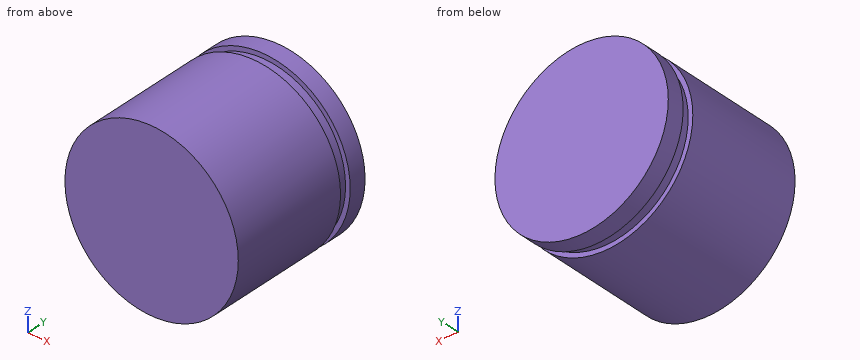
```python
from build123d import *

# Parameters (mm, degrees)
SKETCH1_R           = 7.5
BOSS_EXTRUDE1_DEPTH = 13
SKETCH2_R           = 7.0993
CUT_EXTRUDE1_DEPTH  = 0.9906


with BuildPart() as part:
    # Sketch1 → Boss-Extrude1 (new body)
    with BuildSketch(Plane(origin=(0, 0, 0), x_dir=(1, 0, 0), z_dir=(0, 1, 0))):
        Circle(SKETCH1_R)
    extrude(amount=BOSS_EXTRUDE1_DEPTH)

    # Sketch2 → Cut-Extrude1 (cut)
    with BuildSketch(Plane(origin=(0, 11.476, 0), x_dir=(1, 0, 0), z_dir=(0, 1, 0))):
        Polygon((-10.537332024, 10.483478538), (-10.860452938, -10.950208747), (14.271173695, -10.950208747), (12.440155183, 11.524645927), align=None)
        Circle(SKETCH2_R, mode=Mode.SUBTRACT)
    extrude(amount=-CUT_EXTRUDE1_DEPTH, mode=Mode.SUBTRACT)


solid = part.part
```
Read the model definition and answer for the solid it produces. Units are mm, in the model's axes. Coordinates: 2 decimals unless noted, no trailing zeros. Loops run counter-clockwise (first coordinate to the right, second up) from the corner with the lowest first, then second, coordinate; pieces in that order, holes last.
(1) Flat-ended cylindrical pins translate along their axes: pin 1 Ø3 at (x, y) = (-3, 2) entering from +Z; pin 2 Ø2 at (x, y) = (5.5, 3.5) entering from +Z; pin 3 Ø1 at (x, z) = (-6, 6) entering from +Y; pin 4 Ø5 at (x, y) = (-3, 4) entering from +Z. Find the tip coordinate at first contact, or state that the pin passes through.
Solution:
pin 1: stops at z = 7.35
pin 2: stops at z = 6
pin 3: passes through
pin 4: stops at z = 7.48
(2) The part is cut by section C-C (y = 12.25). Determine the outline of the cut face in (x, z).
Solution:
outline: circle Ø15 at (0, 0)
(3) Consider line 1 along Y through (x, z) = (-5, -5.5); line 2 along X through (y, z) = (4.75, 0.25); line 3 along Z through (x, y) = (-6, 0.5). Determine where each line is inside the solid, lowest interval first.
Solution:
line 1: y = 0 to 10.49, 11.48 to 13
line 2: x = -7.5 to 7.5
line 3: z = -4.5 to 4.5
(4) The part is cut by section B-B (x = 4). Determine the outline of the cut face in (y, z).
Solution:
outline: (0, -6.34) - (10.49, -6.34) - (10.49, -5.87) - (11.48, -5.87) - (11.48, -6.34) - (13, -6.34) - (13, 6.34) - (11.48, 6.34) - (11.48, 5.87) - (10.49, 5.87) - (10.49, 6.34) - (0, 6.34) - close
(5) The part is cut by section A-A (z = -2.75). Determine the outline of the cut face in (x, y).
Solution:
outline: (-6.98, 0) - (6.98, 0) - (6.98, 10.49) - (6.55, 10.49) - (6.55, 11.48) - (6.98, 11.48) - (6.98, 13) - (-6.98, 13) - (-6.98, 11.48) - (-6.55, 11.48) - (-6.55, 10.49) - (-6.98, 10.49) - close
